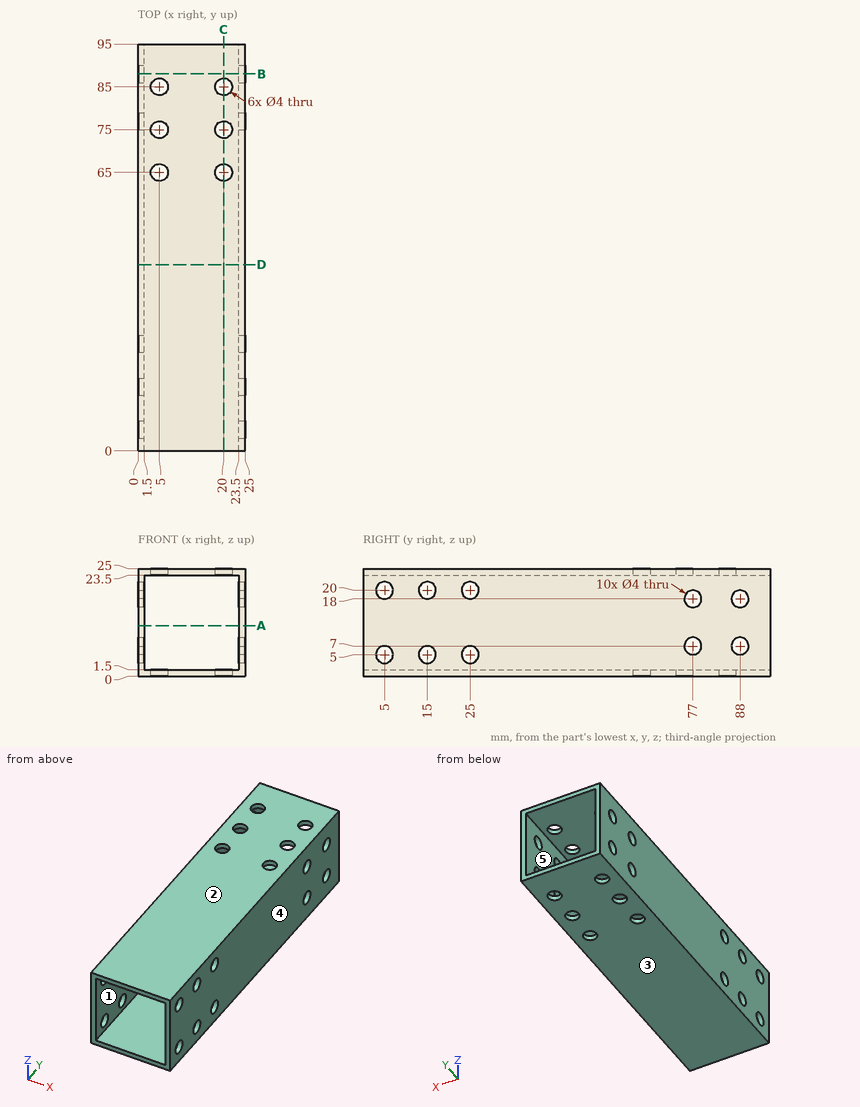
Design review of the part shown in the three views and the two pictorial views. Dimensions are in mm from the part's minimum x, y and z. A direction names the side the tool comes from. Coordinates: 2 decimals unless noted, no trailing zeros. Order: outer loops, then holes, each group sorted by start corner. A loop starts at its lowest first (then second) coordinate and runs counter-clockwise, first axis right, second up. Notation, with made-up numbers: (67.5, 63) - (104.5, 63) arc R22 ccw to (104.5, 77) - close; hole circle Ø6 at (-4, 1.25). An arc over 180 degrees is marked (long way). Answer as CSV lines item,"result". Start each with the question number.
1) Insertion check: P1, Ø3, axis at y = 78.5, z = 12, coming from the -X side. The pin has a flat end and moves straight along its axis. Give the tip position at first contact, or say it passes through.
2) Draft analysis for pull direction Z (two halves, no side actions). For the marked faces 3, 4 and 5, state which applies: +Z half, -Z half, draft (parallel to the pull), parting line (faces both ways), or undercut.
3) To check wall thickness, follow line 1 along Z through (x, y) = (23.95, 88); line 2 along Y through (x, z) = (20, 24); line 3 along X through (y, z) = (57, 16.5). State the ranges of each line that lie inside material, in increasing order. Write a range as [from, to].
4) Add section D-D (y = 43.5). State the section outline as (x, z) points, then the cut area to 3 significant figures.
5) Add section C-C (x = 20). Count the separate pieces of the cut face and the enclosed holes in it, then the cut area to 3 significant figures.
6) Add section B-B (y = 88). State the section outline as (x, z) points, then the cut area to 3 significant figures.
7) Add section A-A (z = 11.75). State the section outline as (x, y) points, then the cut area to 3 significant figures.
8) Machinability: for the marked faces 1 and 2, which of the approach directions +Z, -Z, +X, -X, +Y, -Y give a long, thin tool a straight path to every point of the face, cutting with its end or side? Answer none if there is none.
Result:
1,P1,"x = 0"
2,face 3,"-Z half"
2,face 4,"draft"
2,face 5,"undercut"
3,line 1,"[0, 5], [9, 16], [20, 25]"
3,line 2,"[0, 63], [67, 73], [77, 83], [87, 95]"
3,line 3,"[0, 1.5], [23.5, 25]"
4,outline,"(0, 0) - (25, 0) - (25, 25) - (0, 25) - close; hole (1.5, 1.5) - (23.5, 1.5) - (23.5, 23.5) - (1.5, 23.5) - close"
4,area,"141 mm^2"
5,separate pieces,"8"
5,enclosed holes,"0"
5,area,"249 mm^2"
6,outline,"(0, 0) - (25, 0) - (25, 5) - (23.5, 5) - (23.5, 1.5) - (1.5, 1.5) - (1.5, 5) - (0, 5) - close; (0, 9) - (1.5, 9) - (1.5, 16) - (0, 16) - close; (0, 20) - (1.5, 20) - (1.5, 23.5) - (23.5, 23.5) - (23.5, 20) - (25, 20) - (25, 25) - (0, 25) - close; (23.5, 9) - (25, 9) - (25, 16) - (23.5, 16) - close"
6,area,"117 mm^2"
7,outline,"(0, 0) - (1.5, 0) - (1.5, 95) - (0, 95) - close; (23.5, 0) - (25, 0) - (25, 95) - (23.5, 95) - close"
7,area,"285 mm^2"
8,face 1,"+Y, -Y"
8,face 2,"+Z, +X, -X, +Y, -Y"
